The model under review builds one solid part; all positions refer to its coordinate system, in mm. Round coordinates to 2 decimals unless told otherwise and drop trailing zeros. Loops run counter-clockwise (first coordinate to the right, second up) from the corner with the lowest first, then second, coordinate; pieces in that order, holes last. Notation, with made-up numbers: M 61,-25 L 104,-25 A37 ccw 104,14 Z; hole C 62,0 d5. An arc over 180 degrees is marked long. Answer as a JSON object with one key per item and string values. Group by question number.
Item 1: To check wall thickness, follow line 1 (Z direction, x = 25.5, y = -2); line 2 (X direction, y = 3.5, z = -5.75); line 3 (Z direction, x = 34, y = 3.25). State the ranges of each line that lie inside material, in increasing order.
Item 2: Insertion check: P1, Ø4, axis at x = 56.5, z = -2.5, coming from the -Y side (3 decimals); P2, Ø4, axis at x = 32, z = -1.5, coming from the +Y side; P3, Ø1, axis at x = 51.5, y = 1.5, coming from the -Z side. Each pin has a flat end and moves straight along its axis. Give the tip position at first contact, or say it passes through.
Item 3: Consider section A-A (x = 33). Give the boundary of the cut face in (y, z).
```python
from build123d import *

# Parameters (mm, degrees)
F0_W    = 76.2
F0_H    = 4.826
F2_SIZE = 1.27
F3_SIZE = 1.27


with BuildPart() as f1:
    # F0 (on Front) → F1 (revolve)
    with BuildSketch(Plane.XZ):
        with Locations((38.1, -2.413)):
            Rectangle(F0_W, F0_H)
    revolve(axis=Axis((38.1, 0, -4.826), (1, 0, 0)))

    # F2
    f2_edges = [f1.edges().sort_by_distance(p)[0] for p in [
        (0, 0, -9.652),
    ]]
    chamfer(f2_edges, length=F2_SIZE)

    # F3
    f3_edges = [f1.edges().sort_by_distance(p)[0] for p in [
        (76.2, 0, -9.652),
    ]]
    chamfer(f3_edges, length=F3_SIZE)


solid = f1.part
```
Geometry results:
{
 "1": {"line 1": "z = -9.22 to -0.43", "line 2": "x = 0.06 to 76.14", "line 3": "z = -8.39 to -1.26"},
 "2": {"P1": "stops at y = -4.815", "P2": "stops at y = 4.64", "P3": "stops at z = -9.55"},
 "3": {"outline": "C 0,-4.83 d9.65"}
}
